The listing builds one solid part. Answer for the finished solid, in the listing's coordinates (mm). Face numbers are marked on the shaded views. A direction names the side the tool comes from. Give positions to 0.01 mm unless a question says otherwise; leave off trailing zeros. Write each loop counter-clockwise with the first axis right and the second up, starting at its lowest first coordinate (ties: lowest second). Pieces come first, ordered by that corner, then holes. Notation, with made-up numbers: (41.25, 40.5) -> (56.25, 40.5) arc R31 cw to (56.25, 73.5) -> close; hole circle Ø4 at (-11, 19.25). An arc over 180 degrees is marked (long way). Write each question's results on one line, items separated by ' | '. Start each with the question number.
Autodesk Inventor part; units mm, degrees
ref_plane "YZ Plane" through (0, 0, 0) normal (1, 0, 0) x (0, 1, 0)
ref_plane "XZ Plane" through (0, 0, 0) normal (0, 1, 0) x (-1, 0, 0)
ref_plane "XY Plane" through (0, 0, 0) normal (0, 0, 1) x (1, 0, 0)
sketch "Sketch1" plane through (0, 0, 0) normal (0, 1, 0) x (-1, 0, 0)
  line L0 (72.5, -45) -> (-72.5, -45)
  line L1 (-72.5, -45) -> (-72.5, 45)
  line L2 (-72.5, 45) -> (72.5, 45)
  line L3 (72.5, 45) -> (72.5, -45)
  line L4 (72.5, -45) -> (-72.5, 45) construction
  line L5 (-72.5, -45) -> (72.5, 45) construction
  point P0 (0, 0)
  dimension "d0" = 145
  dimension "d1" = 90
extrude "Extrusion1" add sketch "Sketch1" along normal blind 3
sketch "Sketch4" plane through (72.5, 0, -45) normal (0, 0, -1) x (-1, 0, 0)
  line L0 (35, 3) -> (110, 3)
  line L1 (110, 3) -> (110, -2)
  line L2 (110, -2) -> (35, -2)
  line L3 (35, -2) -> (35, 3)
  line L4 (35, 3) -> (110, -2) construction
  line L5 (110, 3) -> (35, -2) construction
  line L6 (0, 3) -> (145, 3)
  point P0 (72.5, 0)
  point P1 (72.5, 0.5)
  dimension "d28" = 75
  dimension "d29" = 5
  dimension "d30" = 0
extrude "Extrusion3" add sketch "Sketch4" along normal blind 50
sketch "Sketch3" plane through (0, 3, 0) normal (0, 1, 0) x (1, 0, 0)
  circle A0 centre (62.5, -34.9998) radius 2.5
  circle A1 centre (-62.5, -35) radius 2.5
  circle A2 centre (-29.5, 24.592) radius 2.5
  circle A3 centre (29.5, 24.5938) radius 2.5
  line L0 (-72.5, 45) -> (-72.5, -45)
  line L1 (-72.5, -45) -> (72.5, -45)
  point P0 (0, 0)
  dimension "d4" = 5
  dimension "d7" = 5
  dimension "d10" = 5
  dimension "d13" = 5
  dimension "d20" = 59
  dimension "d21" = 125
  dimension "d22" = 33
  dimension "d23" = 59.592
  dimension "d24" = 10
  dimension "d25" = 10
extrude "Extrusion2" cut sketch "Sketch3" against normal through all
properties part number "chasis_arriba"
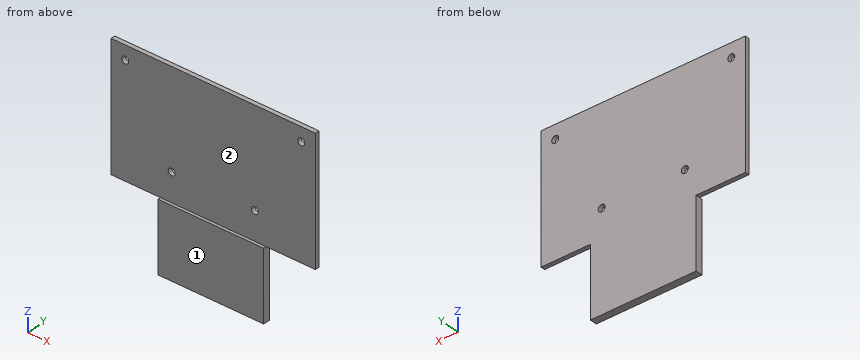
1. Section A-A (x = -29.5) is taken. Write down the section's boundary in (y, z), then the cut area to 3 significant figures.
2. Each of these flat-tipped pins is pushed along its axis until it touches: pin 1 Ø4 at (x, z) = (-29.5, -24.592) entering from +Y; pin 2 Ø1.5 at (y, z) = (0.5, -81) entering from -X; pin 3 Ø1.5 at (x, y) = (52.5, 1) entering from -Z; pin 4 Ø6.5 at (x, z) = (-62.5, 35) entering from -Y. Where does it stop, or does it pass through?
3. A tool of negligible diameter and unlimited length cuts with its end or side. For the marked faces 1 and 2, from which of +Z, -Z, +X, -X, +Y, -Y can it reach the whole face along a straight path? Write none if from no direction.
4. Section D-D (z = -37) is taken. Write down the section's boundary in (x, y), then the cut area to 3 significant figures.
5. Consider probe 1 along Z at (x, y) = (-29.5, 1.2); probe 2 along Y at (x, z) = (-45, -16); probe 3 along Z at (x, y) = (13, -0.4). Determine where each line is inside the solid, lowest interval first. Write a range as [from, to].
6. Section B-B (y = 2) is taken. Write down the section's boundary in (x, z), then the cut area to 3 significant figures.
7. Section C-C (x = 62.5) is taken. Write down the section's boundary in (y, z), then the cut area to 3 significant figures.
Results:
1) outline: (-2, -95) -> (3, -95) -> (3, -27.09) -> (0, -27.09) -> (0, -45) -> (-2, -45) -> close; (0, -22.09) -> (3, -22.09) -> (3, 45) -> (0, 45) -> close | area: 505 mm²
2) pin 1: passes through | pin 2: stops at x = -37.5 | pin 3: stops at z = -45 | pin 4: stops at y = 0
3) face 1: +Z, -Z, +X, -X, -Y | face 2: +Z, +X, -X, -Y
4) outline: (-72.5, 0) -> (72.5, 0) -> (72.5, 3) -> (-72.5, 3) -> close | area: 435 mm²
5) probe 1: z = [-95, -27.09], [-22.09, 45] | probe 2: y = [0, 3] | probe 3: z = [-95, -45]
6) outline: (-72.5, -45) -> (-37.5, -45) -> (-37.5, -95) -> (37.5, -95) -> (37.5, -45) -> (72.5, -45) -> (72.5, 45) -> (-72.5, 45) -> close; hole circle Ø5 at (-62.5, 35); hole circle Ø5 at (-29.5, -24.59); hole circle Ø5 at (29.5, -24.59); hole circle Ø5 at (62.5, 35) | area: 16,700 mm²
7) outline: (0, -45) -> (3, -45) -> (3, 32.5) -> (0, 32.5) -> close; (0, 37.5) -> (3, 37.5) -> (3, 45) -> (0, 45) -> close | area: 255 mm²
